Check sheet for the modelled part. Datum: model origin and axes. Units: mm. A direction names the side the tool comes from. Round coordinates to 2 decimals unless told otherwise and drop trailing zeros. Loops run counter-clockwise (first coordinate to the right, second up) from the corner with the lowest first, then second, coordinate; pieces in that order, holes last. Notation, with made-up numbers: (11.25, 71.25) - (40.25, 71.25) arc R12 ccw to (40.25, 76.25) - close; hole circle Ø1 at (21.25, 35.25). An arc over 180 degrees is marked (long way). Answer in a Markdown table with one row per item. Add a question column.
(1) Thickness scan on line 1 along Y through (x, z) = (5.25, -2.5); line 2 along X through (y, z) = (2, -4.5); line 3 along Y through (x, z) = (-6.25, -8.75). Record the ranges inside material, lowest first.
(2) Cross-section at A-A on z = -14.5. Enter the section's corners in (x, y).
(3) Cross-section at B-B on z = -8.5. Count the separate pieces of the cut face and the enclosed holes in it, then the cut area to 3 significant figures.
(4) Gauge pin test, flat ends, axial feed: pin 1 (1 mm diameter, centred on x = 2.5, y = 6, fed in from +Z); pin 2 (1.7 mm diameter, centred on y = 4.5, z = -4, fed in from -X); pin 3 (4 mm diameter, centred on y = 3.5, z = -5.5, fed in from -X). Record the tip position at first contact, or that the pin passes through.
(5) Mould release check, pull along Z, two halves, no side actions. Record for faces 4 (the flat face through (6.986, 3.944, -5.585)), 5 (the flat face through (-6.45, 4, -1)), 6 (the cylindrical face through (6.25, 2.78, -6.99)), 7 (the cylindrical face through (-6.295, 3.234, -6.733)): +Z half, -Z half, draft (parallel to the pull), parting line (faces both ways), or undercut.
(6) Access from +Z, -Z, +X, -X, +Y, -Y to the whole of each face (thin tool, end or side, straight path). Record for faces 1 (the flat face through (-2.4, 3.1, -13)), 2 (the flat face through (0, 7, 0)), 3 (the flat face through (2.029, 4, -8)).
from build123d import *

# Parameters (mm, degrees)
BOSS_EXTRUDE1_DEPTH     = 8
FILLET1_R               = 0.5
SKETCH5_R               = 2.45
BOSS_EXTRUDE2_DEPTH     = 6
BOSS_EXTRUDE2_TAPER     = 1
CUT_EXTRUDE4_DEPTH      = 2.8
CUT_EXTRUDE4_DEPTH_BACK = 2.8
SKETCH10_R              = 1.45
CUT_EXTRUDE5_DEPTH      = 6
CUT_EXTRUDE5_TAPER      = 1
SKETCH7_R               = 2
CUT_EXTRUDE6_DEPTH      = 1
SKETCH8_R               = 2
CUT_EXTRUDE7_DEPTH      = 1
BOSS_EXTRUDE4_START     = -0.2
SKETCH11_W              = 0.564613496
SKETCH11_H              = 0.366319064
SKETCH11_W_2            = 0.56674541
SKETCH11_H_2            = 0.366442951
BOSS_EXTRUDE4_DEPTH     = 12.3
CUT_EXTRUDE8_DEPTH      = 3
CUT_EXTRUDE8_DEPTH_BACK = 2.5


with BuildPart() as part:
    # Sketch3 → Boss-Extrude1 (new body)
    with BuildSketch(Plane(origin=(0, 0, 0), x_dir=(1, 0, 0), z_dir=(0, 1, 0))):
        Polygon((7.75, 0), (-7.75, 0), (-7.75, 1), (-5.75, 13), (5.75, 13), (7.75, 1), align=None)
    extrude(amount=BOSS_EXTRUDE1_DEPTH)

    # Fillet1
    fillet1_edges = [part.edges().sort_by_distance(p)[0] for p in [
        (5.75, 4, -13),
        (-5.75, 4, -13),
    ]]
    fillet(fillet1_edges, radius=FILLET1_R)

    # Sketch5 → Boss-Extrude2 (add)
    with BuildSketch(Plane(origin=(0, 0, -13), x_dir=(-1, 0, 0), z_dir=(0, 0, -1))):
        with Locations((0, 4.19602759)):
            Circle(SKETCH5_R)
    extrude(amount=BOSS_EXTRUDE2_DEPTH, taper=BOSS_EXTRUDE2_TAPER)

    # Sketch9 → Cut-Extrude4 (cut, two sides)
    with BuildSketch(Plane(origin=(0, 4, 0), x_dir=(1, 0, 0), z_dir=(0, 1, 0))) as cut_extrude4_sk:
        Polygon((-6.45, 0), (-6.45, 2), (-4.95, 11), (-2.467455065, 12), (-1.480633364, 12), (1.480633364, 12), (2.467455065, 12), (5.096667593, 11), (6.45, 2), (6.45, 0), align=None)
    extrude(amount=CUT_EXTRUDE4_DEPTH, mode=Mode.SUBTRACT)
    extrude(cut_extrude4_sk.sketch, amount=-CUT_EXTRUDE4_DEPTH_BACK, mode=Mode.SUBTRACT)

    # Sketch10 → Cut-Extrude5 (cut)
    with BuildSketch(Plane.XY.offset(-12)):
        with Locations((0, 4)):
            Circle(SKETCH10_R)
    extrude(amount=-CUT_EXTRUDE5_DEPTH, taper=CUT_EXTRUDE5_TAPER, mode=Mode.SUBTRACT)

    # Sketch7 → Cut-Extrude6 (cut)
    with BuildSketch(Plane(origin=(7.702702703, 0, -1.283783784), x_dir=(-0.164398987, 0, -0.986393924), z_dir=(0.986393924, 0, -0.164398987))):
        with Locations((7.454263289, 4)):
            Circle(SKETCH7_R)
    extrude(amount=-CUT_EXTRUDE6_DEPTH, mode=Mode.SUBTRACT)

    # Sketch8 → Cut-Extrude7 (cut)
    with BuildSketch(Plane(origin=(-7.702702703, 0, -1.283783784), x_dir=(-0.164398987, 0, 0.986393924), z_dir=(-0.986393924, 0, -0.164398987))):
        with Locations((-7.454263289, 4)):
            Circle(SKETCH8_R)
    extrude(amount=-CUT_EXTRUDE7_DEPTH, mode=Mode.SUBTRACT)

    # Sketch11 → Boss-Extrude4 (add)
    with BuildSketch(Plane.XY.offset(BOSS_EXTRUDE4_START)):
        with BuildLine():
            Line((1.528607349, 5.080212301), (1.528607349, 4))
            Line((1.528607349, 4), (2.028607349, 4))
            Line((2.028607349, 4), (2.028607349, 5.080212301))
            ThreePointArc((2.028607349, 5.080212301), (2.101266499, 5.454430085), (2.308685248, 5.774267176))
            ThreePointArc((2.308685248, 5.774267176), (2.690610434, 6.255141934), (2.973871917, 6.8))
            Line((2.973871917, 6.8), (2.426326427, 6.8))
            ThreePointArc((2.426326427, 6.8), (2.213690864, 6.442234714), (1.948724198, 6.121294613))
            ThreePointArc((1.948724198, 6.121294613), (1.637596075, 5.641538977), (1.528607349, 5.080212301))
        make_face()
        with BuildLine():
            ThreePointArc((1.948724198, 1.878705387), (2.213690864, 1.557765286), (2.426326427, 1.2))
            Line((2.426326427, 1.2), (2.973871917, 1.2))
            ThreePointArc((2.973871917, 1.2), (2.690610434, 1.744858066), (2.308685248, 2.225732824))
            ThreePointArc((2.308685248, 2.225732824), (2.101266499, 2.545569915), (2.028607349, 2.919787699))
            Line((2.028607349, 2.919787699), (2.028607349, 4))
            Line((2.028607349, 4), (1.528607349, 4))
            Line((1.528607349, 4), (1.528607349, 2.919787699))
            ThreePointArc((1.528607349, 2.919787699), (1.637596075, 2.358461023), (1.948724198, 1.878705387))
        make_face()
        with Locations((4, 6.616840468)):
            Rectangle(SKETCH11_W, SKETCH11_H)
        with Locations((4, 1.383221476)):
            Rectangle(SKETCH11_W_2, SKETCH11_H_2)
    boss_extrude4 = extrude(amount=-BOSS_EXTRUDE4_DEPTH)

    # Mirror1: Boss-Extrude4 across plane
    add(boss_extrude4.mirror(Plane(origin=(0, 0, 0), x_dir=(0, 0, 1), z_dir=(1, 0, 0))))

    # Sketch12 → Cut-Extrude8 (cut, two sides)
    with BuildSketch(Plane(origin=(0, 0, 0), x_dir=(0, 0, -1), z_dir=(1, 0, 0))) as cut_extrude8_sk:
        with BuildLine():
            Line((0, 6.910389693), (0, 6.125652773))
            ThreePointArc((0, 6.125652773), (0.255989552, 5.45748479), (0.892896907, 5.131404852))
            Line((0.892896907, 5.131404852), (3.877195183, 4.809928115))
            ThreePointArc((3.877195183, 4.809928115), (4.60456136, 4), (3.877195183, 3.190071885))
            Line((3.877195183, 3.190071885), (0.892896907, 2.868595148))
            ThreePointArc((0.892896907, 2.868595148), (0.255989552, 2.54251521), (0, 1.874347227))
            Line((0, 1.874347227), (0, 1.089610307))
            Line((0, 1.089610307), (-0.964322492, 1.089610307))
            Line((-0.964322492, 1.089610307), (-0.964322492, 6.910389693))
            Line((-0.964322492, 6.910389693), (0, 6.910389693))
        make_face()
    extrude(amount=CUT_EXTRUDE8_DEPTH, mode=Mode.SUBTRACT)
    extrude(cut_extrude8_sk.sketch, amount=-CUT_EXTRUDE8_DEPTH_BACK, mode=Mode.SUBTRACT)


solid = part.part
Answers:
| question | item | result |
|---|---|---|
| 1 | line 1 | y = 0 to 1.2, 6.8 to 8 |
| 1 | line 2 | x = -7.17 to -6.03, -2.51 to -1.84, 1.84 to 2.51, 6.07 to 7.17 |
| 1 | line 3 | y = 0 to 2.01, 5.99 to 8 |
| 2 | outline | circle Ø4.85 at (0, 4.2); hole circle Ø2.81 at (0, 4) |
| 3 | separate pieces | 1 |
| 3 | enclosed holes | 3 |
| 3 | area | 42.2 mm^2 |
| 4 | pin 1 | stops at z = -0.2 |
| 4 | pin 2 | stops at x = -7.39 |
| 4 | pin 3 | stops at x = -7.33 |
| 5 | face 4 | -Z half |
| 5 | face 5 | draft |
| 5 | face 6 | undercut |
| 5 | face 7 | undercut |
| 6 | face 1 | -Z |
| 6 | face 2 | +Z, +X, -X, +Y, -Y |
| 6 | face 3 | +Z |
